Design review of the part built by this model. Coordinates are the model's own, in mm. A direction names the side the tool comes from. Coordinates: 2 decimals unless noted, no trailing zeros. Loops run counter-clockwise (first coordinate to the right, second up) from the corner with the lowest first, then second, coordinate; pieces in that order, holes last. Notation, with made-up numbers: M 43.25,-8.5 L 79.25,-8.5 A17 ccw 79.25,17.5 Z; hole C 27,15.5 d9. An arc over 180 degrees is marked long. Answer as a JSON object with one key per item and string values. Group by question number.
1. Consider section D-D (y = 5.25). State the section outline as (x, z) points.
2. Insertion check: pin 1 (1 mm diameter, centred on y = 6, z = 2, fed in from -X); pin 2 (0.6 mm diameter, centred on y = 6, z = 2.5, fed in from +X). Each pin has a flat end and moves straight along its axis. Give the tip position at first contact, or say it passes through.
3. Consider section A-A (z = 1.75). State the section outline as (x, y) points, then the cut area to 3 significant figures.
4. Consider section B-B (y = 9.25). State the section outline as (x, z) points.
5. Consider section C-C (x = -0.5). State the section outline as (y, z) points, then the cut area to 3 significant figures.
6. Machinability: for faces 1 (the flat face through (0, 1, 0)), 2 (the flat face through (-1.5, 6, 2)), 3 (the flat face through (1.5, 6, 2)), which of the approach directions +Z, -Z, +X, -X, +Y, -Y give a long, thin tool a straight path to every point of the face, cutting with its end or side? Answer none if there is none.
7. To check wall thickness, follow probe 1 along X at (y, z) = (6.75, 2); probe 2 along X at (y, z) = (7.5, 1.6); probe 3 along X at (y, z) = (3.5, 2). State the ranges of each line that lie inside material, in increasing order.
from build123d import *

# Parameters (mm, degrees)
BOSS_EXTRUDE1_DEPTH = 3.5
SKETCH2_R           = 0.25
BOSS_EXTRUDE2_DEPTH = 3.5


with BuildPart() as part:
    # Sketch1 → Boss-Extrude1 (new body)
    with BuildSketch(Plane.XY):
        with BuildLine():
            Line((-1.5, 4.769696007), (-1.5, 6.8))
            Line((-1.5, 6.8), (1.5, 6.8))
            Line((1.5, 6.8), (1.5, 4.769696007))
            ThreePointArc((1.5, 4.769696007), (0, -5), (-1.5, 4.769696007))
        make_face()
    extrude(amount=BOSS_EXTRUDE1_DEPTH)

    # Sketch2 → Boss-Extrude2 (add)
    with BuildSketch(Plane(origin=(0, 6.8, 0), x_dir=(1, 0, 0), z_dir=(0, 1, 0))):
        with Locations(Location((-0.5, -1.75, 0), (0, 0, 90))):
            Circle(SKETCH2_R)
        with Locations(Location((0.5, -1.75, 0), (0, 0, 90))):
            Circle(SKETCH2_R)
    extrude(amount=BOSS_EXTRUDE2_DEPTH)


solid = part.part
Findings below:
{
 "1": {"outline": "M -1.5,0 L 1.5,0 L 1.5,3.5 L -1.5,3.5 Z"},
 "2": {"pin 1": "stops at x = -1.5", "pin 2": "stops at x = 1.5"},
 "3": {"outline": "M -1.5,4.77 A5 ccw long 1.5,4.77 L 1.5,6.8 L 0.75,6.8 L 0.75,10.3 L 0.25,10.3 L 0.25,6.8 L -0.25,6.8 L -0.25,10.3 L -0.75,10.3 L -0.75,6.8 L -1.5,6.8 Z", "area": "87.7 mm^2"},
 "4": {"outline": "C -0.5,1.75 d0.5; C 0.5,1.75 d0.5"},
 "5": {"outline": "M -4.97,0 L 6.8,0 L 6.8,1.5 L 10.3,1.5 L 10.3,2 L 6.8,2 L 6.8,3.5 L -4.97,3.5 Z", "area": "43.0 mm^2"},
 "6": {"face 1": "-Z, +X, -X, +Y, -Y", "face 2": "+Z, -Z, -X, +Y", "face 3": "+Z, -Z, +X, +Y"},
 "7": {"probe 1": "x = -1.5 to 1.5", "probe 2": "x = -0.7 to -0.3, 0.3 to 0.7", "probe 3": "x = -3.57 to 3.57"}
}
